from build123d import *

# Parameters (mm, degrees)
SKETCH1_W           = 77
SKETCH1_H           = 55
BOSS_EXTRUDE1_DEPTH = 27
FILLET1_R           = 10
BOSS_EXTRUDE2_START = -44.75
BOSS_EXTRUDE2_DEPTH = 12.5
SKETCH3_R           = 7.75
CUT_EXTRUDE1_DEPTH  = 12.5


with BuildPart() as part:
    # Sketch1 → Boss-Extrude1 (new body)
    with BuildSketch(Plane.XY):
        with Locations((-38.5, 27.5)):
            Rectangle(SKETCH1_W, SKETCH1_H)
    extrude(amount=BOSS_EXTRUDE1_DEPTH)

    # Fillet1
    fillet1_edges = [part.edges().sort_by_distance(p)[0] for p in [
        (0, 0, 13.5),
        (-77, 0, 13.5),
        (-77, 55, 13.5),
        (0, 55, 13.5),
    ]]
    fillet(fillet1_edges, radius=FILLET1_R)

    # Sketch2 → Boss-Extrude2 (add)
    with BuildSketch(Plane(origin=(0, 0, 0), x_dir=(0, 0, -1), z_dir=(1, 0, 0)).offset(BOSS_EXTRUDE2_START)):
        with BuildLine():
            Line((-2, 0), (-2, -11))
            ThreePointArc((-2, -11), (-2.838969197, -16.434369418), (-8.308548919, -17))
            Line((-8.308548919, -17), (-19, -17))
            ThreePointArc((-19, -17), (-18.23654946, -11.299122875), (-16, -6))
            Line((-16, -6), (-16, 0))
            Line((-16, 0), (-2, 0))
        make_face()
        with BuildLine():
            Line((-4.740210034, -11.700555844), (-4.740210034, -14.646739817))
            ThreePointArc((-4.740210034, -14.646739817), (-7.840210034, -13.17364783), (-4.740210034, -11.700555844))
        make_face(mode=Mode.SUBTRACT)
    extrude(amount=BOSS_EXTRUDE2_DEPTH)

    # Sketch3 → Cut-Extrude1 (cut)
    with BuildSketch(Plane.XY.offset(27)):
        with Locations((-57, 27.5)):
            Circle(SKETCH3_R)
    extrude(amount=-CUT_EXTRUDE1_DEPTH, mode=Mode.SUBTRACT)


solid = part.part
The listing builds one solid part. Answer for the finished solid, in the listing's coordinates (mm). A direction names the side the tool comes from. Round coordinates to 2 decimals unless told otherwise and drop trailing zeros. Order: outer loops, then holes, each group sorted by start corner. A loop starts at its lowest first (then second) coordinate and runs counter-clockwise, first axis right, second up. Notation, with made-up numbers: (88.5, -19) - (125.5, -19) arc R34 cw to (125.5, 16) - close; hole circle Ø7 at (21.25, 36.25). An arc over 180 degrees is marked (long way). Write item = value, one per line. Start each with the question number.
1) Given pin 1 (8 mm diameter, centred on x = -59, y = 25, fed in from +Z); pin 2 (1 mm diameter, centred on x = -60.5, z = 15.5, fed in from -Y); pin 3 (5.5 mm diameter, centred on y = -10.5, z = 14, fed in from +X), each flat-ended and moving along its own axis, determine where each tip first touches the part or whether it passes through.
2) For faces 4 (the cylindrical face through (-38.59, -11.38, 18.26)), 5 (the flat face through (-44.75, -9, 10)), 6 (the flat face through (-57, 28, 14.5)), 7 (the flat face through (-32.25, -9, 10)), determine the directions among +Z, -Z, +X, -X, +Y, -Y from which every point of the face is accessible in a straight line to the end or side of a thin tool.
3) Straight lines are drawn through the part: L1, parallel to Y at x = -57, z = 24.5; L2, parallel to Z at x = -37, y = -4.5; L3, parallel to Y at x = -67, z = 23.5. For each, find the intervals that lie inside material, in ascending order.
4) Section C-C, the plane y = 27.5 is taken. Write down the section's boundary in (x, z), plus the area to 3 significant figures.
5) Section A-A, the plane z = 24.75 is taken. Write down the section's boundary in (x, y), plus the area to 3 significant figures.
6) Section D-D, the plane z = 6 is taken. Write down the section's boundary in (x, y).
7) Section B-B, the plane x = -39.5 is taken. Write down the section's boundary in (y, z).
8) For a pull along Z with two mould halves and no side action, classify faces 1 (the cylindrical face through (-3.01, 2.85, 13.69)), 2 (the flat face through (-39, -5, 2)), 3 (the cylindrical face through (-38.59, -13.23, 7.84)) as released by +Z, released by -Z, zero draft, split by the parting line, or undercut.
Results list:
q1.pin_1 = 14.5
q1.pin_2 = 0
q1.pin_3 = -32.25
q2.face_4 = +Z, +X, -X
q2.face_5 = +Z, -Z, -X, -Y
q2.face_6 = +Z
q2.face_7 = +Z, -Z, +X, -Y
q3.L1 = 0 to 19.75, 35.25 to 55
q3.L2 = 2 to 16
q3.L3 = 0 to 55
q4.outline = (-77, 0) - (0, 0) - (0, 27) - (-49.25, 27) - (-49.25, 14.5) - (-64.75, 14.5) - (-64.75, 27) - (-77, 27) - close
q4.area = 1,890 mm^2
q5.outline = (-77, 10) arc R10 ccw to (-67, 0) - (-10, 0) arc R10 ccw to (0, 10) - (0, 45) arc R10 ccw to (-10, 55) - (-67, 55) arc R10 ccw to (-77, 45) - close; hole circle Ø15.5 at (-57, 27.5)
q5.area = 3,960 mm^2
q6.outline = (-77, 10) arc R10 ccw to (-67, 0) - (-44.75, 0) - (-44.75, -11.27) - (-32.25, -11.27) - (-32.25, 0) - (-10, 0) arc R10 ccw to (0, 10) - (0, 45) arc R10 ccw to (-10, 55) - (-67, 55) arc R10 ccw to (-77, 45) - close; (-44.75, -17.67) - (-32.25, -17.67) - (-32.25, -15.07) - (-44.75, -15.07) - close
q7.outline = (-17, 8.31) arc R4.5 ccw to (-11, 2) - (0, 2) - (0, 0) - (55, 0) - (55, 27) - (0, 27) - (0, 16) - (-6, 16) arc R21.67 ccw to (-17, 19) - close; hole (-14.65, 4.74) - (-11.7, 4.74) arc R1.9 ccw (long way) to start
q8.face_1 = zero draft
q8.face_2 = released by -Z
q8.face_3 = undercut
